from build123d import *

# Parameters (mm, degrees)
HEX_2_DEPTH = 2


with BuildPart() as part:
    # Threads_Sketch → Threads (revolve)
    with BuildSketch(Plane.XY, mode=Mode.PRIVATE) as threads_sk:
        Polygon((0, 0), (0, 4.958321687), (7, 4.740416799), (7, 0), align=None)
    revolve(threads_sk.sketch.rotate(Axis((-5.91867895, 0, 0), (1, 0, 0)), 90), axis=Axis((-5.91867895, 0, 0), (1, 0, 0)))

    # Threads Cham: read off the stored shape, not the designer's step
    # Threads Cham outline → Threads Cham (revolve, cut)
    with BuildSketch(Plane.YX):
        Polygon((4.160416799, 7), (4.759051872, 6.401364927), (4.759051872, 7), align=None)
        Polygon((4.940275453, 0), (4.940275453, 0.579719185), (4.395559124, 0), align=None)
    revolve(axis=Axis((0, 0, 0), (1, 0, 0)), mode=Mode.SUBTRACT)

    # Threads Cham 2 outline → Threads Cham 2 (revolve, cut)
    with BuildSketch(Plane.YX):
        Polygon((4.940275453, 0.579719185), (4.940275453, 0), (4.958321687, 0), align=None)
    revolve(axis=Axis((0, 0, 0), (1, 0, 0)), mode=Mode.SUBTRACT)

    # Hex_Sketch → Hex 2 (cut)
    with BuildSketch(Plane.ZY):
        Polygon((2.748187281, 0), (1.374093641, 2.38), (-1.374093641, 2.38), (-2.748187281, 0), (-1.374093641, -2.38), (1.374093641, -2.38), align=None)
    extrude(amount=-HEX_2_DEPTH, mode=Mode.SUBTRACT)


solid = part.part
The listing builds one solid part. Answer for the finished solid, in the listing's coordinates (mm). A direction names the side the tool comes from. Give positions to 0.01 mm unless a question says otherwise; leave off trailing zeros. Write each loop counter-clockwise with the first axis right and the second up, starting at its lowest first coordinate (ties: lowest second). Pieces come first, ordered by that corner, then holes. Notation, with made-up numbers: (-36, 30) - (-9, 30) arc R8 cw to (-9, 41) - close; hole circle Ø10 at (-2.75, 76). An arc over 180 degrees is marked (long way). One line per question, with ' | ' between items. Start each with the question number.
1. For faces 1 (the face through (0, 2, -2)), 2 (the face through (0.986, -1.173, -2.071)), determine the directions among +Z, -Z, +X, -X, +Y, -Y from which every point of the face is accessible in a straight line to the end or side of a thin tool.
2. Straight lines are drawn through the part: line 1 (X direction, y = -0.25, z = -2.5); line 2 (Z direction, x = 1.25, y = -1.25); line 3 (Z direction, x = 0.5, y = 0.5). For each, find the intervals that lie inside material, in ascending order.
3. Section A-A, the plane x = 1.25 is taken. Determine the outline of the cut face in (y, z), then the cut area to 3 significant figures.
4. Section D-D, the plane x = 4 is taken. Determine the outline of the cut face in (y, z), then the cut area to 3 significant figures.
5. Section B-B, the plane z = 0 is taken. Determine the outline of the cut face in (x, y), then the cut area to 3 significant figures.
6. Given P1, Ø1.6, axis at x = 1.5, z = 0, coming from the +Y side; P2, Ø2, axis at y = 3.5, z = -4, coming from the +X side; P3, Ø4, axis at x = 2, y = 4, coming from the -Z side, each flat-ended and moving along its own axis, determine where each tip first touches the part or whether it passes through.
7. Section C-C, the plane x = 5.5 is taken. Determine the outline of the cut face in (y, z), then the cut area to 3 significant figures.
8. Determine the mould class of faces 3 (the face through (0.986, 1.173, 2.071)), 4 (the face through (3.531, -1.456, 4.625)), 5 (the face through (7, 0, 0)), 6 (the face through (0.99, 1.21, -2.05)) for opening direction Z: +Z half, -Z half, draft (parallel to the pull), parting line (faces both ways), or undercut.
Result:
1) face 1: +Z, -Z, -X, +Y, -Y | face 2: -X
2) line 1: x = 2 to 7 | line 2: z = -4.76 to -2.03, 2.03 to 4.76 | line 3: z = -4.84 to -2.46, 2.46 to 4.84
3) outline: circle Ø9.84 at (0, 0); hole (-2.38, -1.37) - (0, -2.75) - (2.38, -1.37) - (2.38, 1.37) - (0, 2.75) - (-2.38, 1.37) - close | area: 56.4 mm2
4) outline: circle Ø9.67 at (0, 0) | area: 73.4 mm2
5) outline: (0, -4.4) - (0.58, -4.94) - (6.4, -4.76) - (7, -4.16) - (7, 4.16) - (6.4, 4.76) - (0.58, 4.94) - (0, 4.4) - (0, 2.38) - (2, 2.38) - (2, -2.38) - (0, -2.38) - close | area: 57.7 mm2
6) P1: stops at y = 4.94 | P2: stops at x = 6.85 | P3: stops at z = -4.47
7) outline: circle Ø9.57 at (0, 0) | area: 72.0 mm2
8) face 3: undercut | face 4: parting line | face 5: draft | face 6: undercut
